Check sheet for the modelled part. Datum: model origin and axes. Units: mm. Face numbers are marked on the shaded views. A direction names the side the tool comes from. Round coordinates to 2 decimals unless told otherwise and drop trailing zeros. Write each loop counter-clockwise with the first axis right and the second up, starting at its lowest first coordinate (ties: lowest second). Pieces come first, ordered by that corner, then holes.
Item 1: Section check A-A, the plane y = 7.25. Record the cut outline in (x, z), plus the area to 3 significant figures.
Item 2: Release check for a two-part mould opening along X. For the marked faces 1, 2, 3 and 4 record: pulls with the +X half, pulls with the -X half, needs draft (parallel to the pull), parting line crosses it, or undercut.
Item 3: Section check B-B, the plane z = 7. Record the cut outline in (x, y).
Item 4: Set-up check for the marked faces 5 and 6: record each of +Z, -Z, +X, -X, +Y, -Y from which the full face is reachable in a straight line by a thin tool's end or side.
Item 5: Material ranges on line 1 along X through (y, z) = (7, 46.5); line 2 along Z through (x, y) = (-78.5, 4.75); line 3 along Y through (x, z) = (-75, 19), recorded low to high.
Item 6: Section check C-C, the plane x = -83.5. Record the cut outline in (y, z), plus the area to 3 significant figures.
Item 7: Depth check by flat-ended pin: pin 1 (1.5 mm diameter, centred on x = -109.5, z = 46, fed in from +Y). Enter the tip coordinate at first touch or a pass-through.
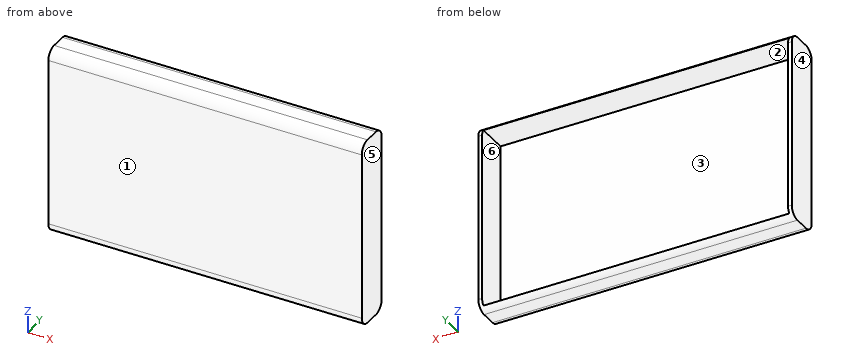
Autodesk Inventor part; units mm, degrees
ref_plane "YZ Plane" through (0, 0, 0) normal (1, 0, 0) x (0, 1, 0)
ref_plane "XZ Plane" through (0, 0, 0) normal (0, 1, 0) x (-1, 0, 0)
ref_plane "XY Plane" through (0, 0, 0) normal (0, 0, 1) x (1, 0, 0)
sketch "Sketch1" plane through (0, 0, 0) normal (0, 1, 0) x (-1, 0, 0)
  line L0 (0, 0) -> (125, 0)
  line L1 (125, 0) -> (125, 75)
  line L2 (125, 75) -> (0, 75)
  line L3 (0, 75) -> (0, 0)
  dimension "d0" = 125
  dimension "d1" = 75
extrude "Extrusion1" add sketch "Sketch1" along normal blind 1
sketch "Sketch2" plane through (0, 1, 0) normal (0, 1, 0) x (1, 0, 0)
  point P0 (0, 0)
sketch "Sketch3" plane through (0, 1, 0) normal (0, 1, 0) x (1, 0, 0)
  point P0 (0, 0)
sketch "Sketch4" plane through (0, 1, 0) normal (0, 1, 0) x (1, 0, 0)
  line L0 (-125, -75) -> (0, -75)
  line L1 (-125, -75) -> (0, -75)
  line L2 (0, -75) -> (0, 0)
  line L3 (0, 0) -> (-125, 0)
  line L4 (-125, 0) -> (-125, -75)
  line L5 (-123.5, -73.5) -> (-1.5, -73.5)
  line L6 (-1.5, -73.5) -> (-1.5, -1.5)
  line L7 (-1.5, -1.5) -> (-123.5, -1.5)
  line L8 (-123.5, -1.5) -> (-123.5, -73.5)
  dimension "d4" = 1.5
  dimension "d5" = 1.5
  dimension "d6" = 122
  dimension "d7" = 72
extrude "Extrusion2" add sketch "Sketch4" along normal blind 13
fillet "Fillet1" radius 4 1 edges at (-62.5, 14, 75)
fillet "Fillet2" radius 4 1 edges at (-62.5, 14, 0)
fillet "Fillet3" radius 4 1 edges at (-62.5, 0, 75)
fillet "Fillet4" radius 4 1 edges at (-62.5, 0, 0)
properties part number "Raspberry Pi Phone Test"
Values found:
1. outline: (-125, 0) - (0, 0) - (0, 75) - (-125, 75) - close; hole (-123.5, 1.5) - (-1.5, 1.5) - (-1.5, 73.5) - (-123.5, 73.5) - close
1. area: 591 mm2
2. face 1: needs draft
2. face 2: undercut
2. face 3: undercut
2. face 4: pulls with the -X half
3. outline: (-125, 0) - (0, 0) - (0, 14) - (-1.5, 14) - (-1.5, 1) - (-123.5, 1) - (-123.5, 14) - (-125, 14) - close
4. face 5: +Z, -Z, +X, +Y, -Y
4. face 6: +Y
5. line 1: x = -125 to -123.5, -1.5 to 0
5. line 2: z = 0 to 1.5, 73.5 to 75
5. line 3: y = 0 to 1
6. outline: (0, 4) arc R4 ccw to (4, 0) - (10, 0) arc R4 ccw to (13.12, 1.5) - (1, 1.5) - (1, 73.5) - (13.12, 73.5) arc R4 ccw to (10, 75) - (4, 75) arc R4 ccw to (0, 71) - close
6. area: 102 mm2
7. pin 1: stops at y = 1
